Verification items for the finished model (mm, model axes). Face numbers are marked on the shaded views. Give positions to 0.01 mm unless a question says otherwise; leave off trailing zeros. Loops run counter-clockwise (first coordinate to the right, second up) from the corner with the lowest first, then second, coordinate; pieces in that order, holes last. Notation, with made-up numbers: (74.5, 12) - (118.5, 12) arc R19 cw to (118.5, 26) - close; hole circle Ø3 at (26, -32). An arc over 180 degrees is marked (long way). One line per item, written item: value. Start each with the question number.
1. Gauge pin test, flat ends, axial feed: pin 1 (2 mm diameter, centred on x = 25, y = 0.5, fed in from +Z); pin 2 (0.8 mm diameter, centred on x = -47.5, z = 0, fed in from +Y); pin 3 (1.5 mm diameter, centred on y = 3, z = -4, fed in from -X). Record the tip position at first contact, or that the pin passes through.
2. Sectioned sample at A-A (x = 0). Record the cut outline in (y, z), plus the area to 3 significant figures.
3. Sectioned sample at B-B (z = 0). Record the cut outline in (x, y).
4. Mould release check, pull along Y, two halves, no side actions. Record for the marked faces 1 and 2: pulls with the +Y half, pulls with the -Y half, needs draft (parallel to the pull), parting line crosses it, or undercut.
5. Scan lines: L1, parallel to X at y = 2.2, z = 0; L2, parallel to X at y = 0.85, z = 9.5; L3, parallel to Z at x = 15, y = 0.6. Record each from-to range of solid material in increasing order. Write a range as [from, to].
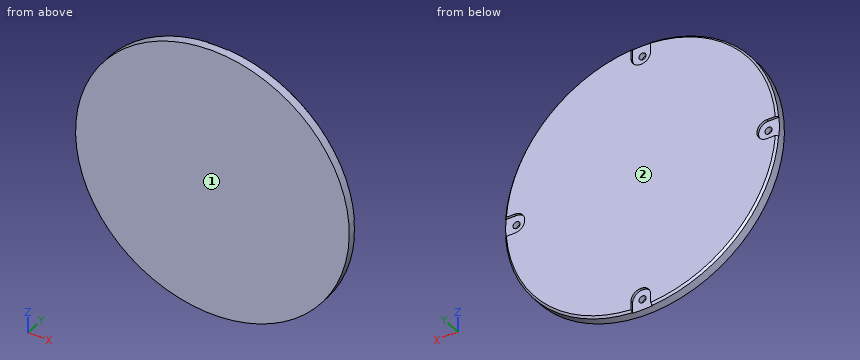
from build123d import *

# Parameters (mm, degrees)
SKETCH1_R           = 52
BOSS_EXTRUDE1_DEPTH = 4
SKETCH2_R           = 1.35
CUT_EXTRUDE2_DEPTH  = 3
CHAMFER1_SIZE       = 0.75
SKETCH3_R           = 1.35
CUT_EXTRUDE3_DEPTH  = 1


with BuildPart() as part:
    # Sketch1 → Boss-Extrude1 (new body)
    with BuildSketch(Plane(origin=(0, 0, 0), x_dir=(1, 0, 0), z_dir=(0, 1, 0))):
        with Locations(Location((0, 0, 0), (0, 0, 270))):
            Circle(SKETCH1_R)
    extrude(amount=BOSS_EXTRUDE1_DEPTH)

    # Sketch2 → Cut-Extrude2 (cut)
    with BuildSketch(Plane(origin=(0, 4, 0), x_dir=(1, 0, 0), z_dir=(0, 1, 0))):
        with Locations(Location((0, 47.88, 0), (0, 0, 270))):
            Circle(SKETCH2_R)
        with Locations(Location((47.88, 0, 0), (0, 0, 270))):
            Circle(SKETCH2_R)
        with Locations(Location((0, -47.88, 0), (0, 0, 270))):
            Circle(SKETCH2_R)
        with Locations(Location((-47.88, 0, 0), (0, 0, 270))):
            Circle(SKETCH2_R)
    extrude(amount=-CUT_EXTRUDE2_DEPTH, mode=Mode.SUBTRACT)

    # Chamfer1
    chamfer1_edges = [part.edges().sort_by_distance(p)[0] for p in [
        (0, 4, -52),
    ]]
    chamfer(chamfer1_edges, length=CHAMFER1_SIZE)

    # Sketch3 → Cut-Extrude3 (cut)
    # profile 1 of 8: a face of its own
    with BuildSketch(Plane(origin=(0, 4, 0), x_dir=(1, 0, 0), z_dir=(0, 1, 0))):
        with BuildLine():
            ThreePointArc((3.75, 51.112620751), (0, 51.25), (-3.75, 51.112620751))
            Line((-3.75, 51.112620751), (-3.75, 47.88))
            ThreePointArc((-3.75, 47.88), (0, 44.13), (3.75, 47.88))
            Line((3.75, 47.88), (3.75, 51.112620751))
        make_face()
        with Locations(Location((0, 47.88, 0), (0, 0, 270))):
            Circle(SKETCH3_R, mode=Mode.SUBTRACT)
    # profile 2 of 8: a face of its own
    with BuildSketch(Plane(origin=(0, 4, 0), x_dir=(1, 0, 0), z_dir=(0, 1, 0))):
        with BuildLine():
            Line((-47.88, 3.75), (-51.112620751, 3.75))
            ThreePointArc((-51.112620751, 3.75), (-51.25, 0), (-51.112620751, -3.75))
            Line((-51.112620751, -3.75), (-47.88, -3.75))
            ThreePointArc((-47.88, -3.75), (-44.13, 0), (-47.88, 3.75))
        make_face()
        with Locations(Location((-47.88, 0, 0), (0, 0, 270))):
            Circle(SKETCH3_R, mode=Mode.SUBTRACT)
    # profile 3 of 8: a face of its own
    with BuildSketch(Plane(origin=(0, 4, 0), x_dir=(1, 0, 0), z_dir=(0, 1, 0))):
        with BuildLine():
            ThreePointArc((51.25, 0), (51.215643672, 1.876257782), (51.112620751, 3.75))
            Line((51.112620751, 3.75), (47.88, 3.75))
            ThreePointArc((47.88, 3.75), (44.13, 0), (47.88, -3.75))
            Line((47.88, -3.75), (51.112620751, -3.75))
            ThreePointArc((51.112620751, -3.75), (51.215643672, -1.876257782), (51.25, 0))
        make_face()
        with Locations(Location((47.88, 0, 0), (0, 0, 270))):
            Circle(SKETCH3_R, mode=Mode.SUBTRACT)
    # profile 4 of 8: a face of its own
    with BuildSketch(Plane(origin=(0, 4, 0), x_dir=(1, 0, 0), z_dir=(0, 1, 0))):
        with BuildLine():
            ThreePointArc((3.75, 51.864607393), (0, 52), (-3.75, 51.864607393))
            Line((-3.75, 51.864607393), (-3.75, 51.112620751))
            ThreePointArc((-3.75, 51.112620751), (0, 51.25), (3.75, 51.112620751))
            Line((3.75, 51.112620751), (3.75, 51.864607393))
        make_face()
    # profile 5 of 8: a face of its own
    with BuildSketch(Plane(origin=(0, 4, 0), x_dir=(1, 0, 0), z_dir=(0, 1, 0))):
        with BuildLine():
            ThreePointArc((-51.112620751, -3.75), (-51.25, 0), (-51.112620751, 3.75))
            Line((-51.112620751, 3.75), (-51.864607393, 3.75))
            ThreePointArc((-51.864607393, 3.75), (-52, 0), (-51.864607393, -3.75))
            Line((-51.864607393, -3.75), (-51.112620751, -3.75))
        make_face()
    # profile 6 of 8: a face of its own
    with BuildSketch(Plane(origin=(0, 4, 0), x_dir=(1, 0, 0), z_dir=(0, 1, 0))):
        with BuildLine():
            Line((51.864607393, 3.75), (51.112620751, 3.75))
            ThreePointArc((51.112620751, 3.75), (51.215643672, 1.876257782), (51.25, 0))
            ThreePointArc((51.25, 0), (51.215643672, -1.876257782), (51.112620751, -3.75))
            Line((51.112620751, -3.75), (51.864607393, -3.75))
            ThreePointArc((51.864607393, -3.75), (52, 0), (51.864607393, 3.75))
        make_face()
    # profile 7 of 8: a face of its own
    with BuildSketch(Plane(origin=(0, 4, 0), x_dir=(1, 0, 0), z_dir=(0, 1, 0))):
        with BuildLine():
            Line((-3.75, -47.88), (-3.75, -51.112620751))
            ThreePointArc((-3.75, -51.112620751), (0, -51.25), (3.75, -51.112620751))
            Line((3.75, -51.112620751), (3.75, -47.88))
            ThreePointArc((3.75, -47.88), (0, -44.13), (-3.75, -47.88))
        make_face()
        with Locations(Location((0, -47.88, 0), (0, 0, 270))):
            Circle(SKETCH3_R, mode=Mode.SUBTRACT)
    # profile 8 of 8: a face of its own
    with BuildSketch(Plane(origin=(0, 4, 0), x_dir=(1, 0, 0), z_dir=(0, 1, 0))):
        with BuildLine():
            ThreePointArc((3.75, -51.112620751), (0, -51.25), (-3.75, -51.112620751))
            Line((-3.75, -51.112620751), (-3.75, -51.864607393))
            ThreePointArc((-3.75, -51.864607393), (0, -52), (3.75, -51.864607393))
            Line((3.75, -51.864607393), (3.75, -51.112620751))
        make_face()
    extrude(amount=-CUT_EXTRUDE3_DEPTH, mode=Mode.SUBTRACT)


solid = part.part
Results are:
1. pin 1: stops at z = 46.13
1. pin 2: stops at y = 1
1. pin 3: stops at x = -51.9
2. outline: (0, -52) - (3, -52) - (3, -49.23) - (1, -49.23) - (1, -46.53) - (3, -46.53) - (3, -44.13) - (4, -44.13) - (4, 44.13) - (3, 44.13) - (3, 46.53) - (1, 46.53) - (1, 49.23) - (3, 49.23) - (3, 52) - (0, 52) - close
2. area: 389 mm^2
3. outline: (-52, 0) - (52, 0) - (52, 3) - (49.23, 3) - (49.23, 1) - (46.53, 1) - (46.53, 3) - (44.13, 3) - (44.13, 4) - (-44.13, 4) - (-44.13, 3) - (-46.53, 3) - (-46.53, 1) - (-49.23, 1) - (-49.23, 3) - (-52, 3) - close
4. face 1: pulls with the -Y half
4. face 2: pulls with the +Y half
5. L1: x = [-52, -49.23], [-46.53, 46.53], [49.23, 52]
5. L2: x = [-51.12, 51.12]
5. L3: z = [-49.79, 49.79]
